```python
from build123d import *


with BuildPart() as part:
    # Sketch1 one side → Revolve1 (revolve)
    with BuildSketch(Plane.XY, mode=Mode.PRIVATE) as revolve1_sk:
        Polygon((-40, 20), (-80, 20), (-80, 0), (0, 0), (35, 0), (80, 0), (80, 20), (40, 20), (40, 40), (25, 40), (25, 35), (-25, 35), (-25, 40), (-40, 40), align=None)
    revolve(revolve1_sk.sketch.rotate(Axis((0, 0, 0), (-1, 0, 0)), 90), axis=Axis((0, 0, 0), (-1, 0, 0)))

    # Sketch1_4 → Revolve3 (revolve)
    with BuildSketch(Plane.XY, mode=Mode.PRIVATE) as revolve3_sk:
        Polygon((0, 80), (0, 35), (25, 35), (25, 40), (20, 40), (20, 80), align=None)
        Polygon((0, 35), (0, 0), (35, 0), (35, 25), (40, 25), (40, 40), (25, 40), (25, 35), align=None)
        Polygon((35, 0), (0, 0), (0, -80), (20, -80), (20, -40), (40, -40), (40, -25), (35, -25), align=None)
    revolve(revolve3_sk.sketch.rotate(Axis((0, 80, 0), (0, -1, 0)), 90), axis=Axis((0, 80, 0), (0, -1, 0)))


solid = part.part
```
The listing builds one solid part. Answer for the finished solid, in the listing's coordinates (mm). A direction names the side the tool comes from. Give positions to 0.01 mm unless a question says otherwise; leave off trailing zeros. Loops run counter-clockwise (first coordinate to the right, second up) from the corner with the lowest first, then second, coordinate; pieces in that order, holes last. Notation, with made-up numbers: M 57,67 L 80,67 A17 ccw 80,73 Z; hole C 44.5,-24 d11. An arc over 180 degrees is marked long. One line per item, written item: value.
Q1. A cutting plane is placed at D-D on z = 3.5. Determine the outline of the cut face in (x, y).
Working result:
outline: M -80,-19.69 L -40,-19.69 L -40,-39.85 L -39.85,-39.85 L -39.85,-40 L -19.69,-40 L -19.69,-80 L 19.69,-80 L 19.69,-40 L 39.85,-40 L 39.85,-39.85 L 40,-39.85 L 40,-19.69 L 80,-19.69 L 80,19.69 L 40,19.69 L 40,39.85 L 39.85,39.85 L 39.85,40 L 19.69,40 L 19.69,80 L -19.69,80 L -19.69,40 L -39.85,40 L -39.85,39.85 L -40,39.85 L -40,19.69 L -80,19.69 Z
Q2. A cutting plane is placed at B-B on y = 38. Determine the outline of the cut face in (x, z), then the cut area to 3 significant figures.
Working result:
outline: M -40,-12.49 L -38,-12.49 A40 ccw 38,-12.49 L 40,-12.49 L 40,12.49 L 38,12.49 A40 ccw -38,12.49 L -40,12.49 Z
area: 5,060 mm^2
Q3. Find the intervals of material crossed by line 1 (X direction, y = 34, z = -17.5); line 2 (Y direction, x = -65, z = 0), in increasing order. Write a range as from..to.
Working result:
line 1: x = -40..40
line 2: y = -20..20
Q4. A cutting plane is placed at A-A on z = -5.5. Determine the outline of the cut face in (x, y).
Working result:
outline: M -80,-19.23 L -40,-19.23 L -40,-39.62 L -39.62,-39.62 L -39.62,-40 L -19.23,-40 L -19.23,-80 L 19.23,-80 L 19.23,-40 L 39.62,-40 L 39.62,-39.62 L 40,-39.62 L 40,-19.23 L 80,-19.23 L 80,19.23 L 40,19.23 L 40,39.62 L 39.62,39.62 L 39.62,40 L 19.23,40 L 19.23,80 L -19.23,80 L -19.23,40 L -39.62,40 L -39.62,39.62 L -40,39.62 L -40,19.23 L -80,19.23 Z
Q5. Flat-ended cylindrical pins translate along their axes: P1, Ø10, axis at x = -56, z = 27, coming from the -Y side; P2, Ø12, axis at y = -45, z = -24.5, coming from the -X side; P3, Ø8, axis at x = -9, z = 31.5, coming from the +Y side; P4, Ø12, axis at x = -15.5, y = -12.5, coming from the +Z side. Find the tip coordinate at first contact, or state that the pin passes through.
Working result:
P1: passes through
P2: stops at x = -33.93
P3: stops at y = 40
P4: stops at z = 34.39
Q6. A cutting plane is placed at C-C on x = 55.5. Determine the outline of the cut face in (y, z).
Working result:
outline: C 0,0 d40
Q7. Determine the mould class of faces 4 (the face through (-60.28, -0.88, 19.98)), 5 (the face through (0, -15, -35)), 6 (the face through (25, 0, -36)), 7 (the face through (-0.88, -59.72, -19.98)) for opening direction X: +X half, -X half, draft (parallel to the pull), parting line (faces both ways), or undercut.
Working result:
face 4: draft
face 5: undercut
face 6: undercut
face 7: parting line
Q8. For faces 1 (the face through (0, 15, -35)), 2 (the face through (40, -18.3, -9.4)), 3 (the face through (-0.88, -32.4, -39.99)), determine the directions among +Z, -Z, +X, -X, +Y, -Y from which every point of the face is accessible in a straight line to the end or side of a thin tool.
Working result:
face 1: -Z
face 2: +X
face 3: -Z, -Y
